from build123d import *

# Parameters (mm, degrees)
F1_DEPTH = 25


with BuildPart() as f1:
    # F0 (on Front) → F1 (new body)
    with BuildSketch(Plane.XZ):
        with BuildLine():
            ThreePointArc((0.492404, 26.751671), (0, 27.164847), (-0.492404, 26.751671))
            Line((-0.492404, 26.751671), (-4.482871, 4.120605))
            ThreePointArc((-4.482871, 4.120605), (-4.605972, 4.017311), (-4.729073, 4.120605))
            Line((-4.729073, 4.120605), (-8.719541, 26.751671))
            ThreePointArc((-8.719541, 26.751671), (-9.211945, 27.164847), (-9.704349, 26.751671))
            Line((-9.704349, 26.751671), (-14.42139, 0))
            Line((-14.42139, 0), (-13.451544, 0))
            Line((-13.451544, 0), (-9.365199, 23.17481))
            ThreePointArc((-9.365199, 23.17481), (-9.242099, 23.278104), (-9.118998, 23.17481))
            Line((-9.118998, 23.17481), (-5.109237, 0.434329))
            ThreePointArc((-5.109237, 0.434329), (-4.945978, 0.126497), (-4.621282, 5.9e-05))
            ThreePointArc((-4.621282, 5.9e-05), (-4.304656, 0.119468), (-4.136591, 0.413176))
            Line((-4.136591, 0.413176), (-4.105972, 0.586824))
            Line((-4.105972, 0.586824), (-0.123101, 23.17481))
            ThreePointArc((-0.123101, 23.17481), (0, 23.278104), (0.123101, 23.17481))
            Line((0.123101, 23.17481), (4.209445, 0))
            Line((4.209445, 0), (5.209445, 0))
            Line((5.209445, 0), (0.492404, 26.751671))
        make_face()
    extrude(amount=F1_DEPTH)


solid = f1.part
The model under review builds one solid part; all positions refer to its coordinate system, in mm. A direction names the side the tool comes from. Coordinates: 2 decimals unless noted, no trailing zeros. Loops run counter-clockwise (first coordinate to the right, second up) from the corner with the lowest first, then second, coordinate; pieces in that order, holes last. Notation, with made-up numbers: (-14, -15.75) -> (18, -15.75) arc R16 cw to (18, 0.25) -> close; hole circle Ø9 at (31, 59.25). An arc over 180 degrees is marked (long way). Use a Markdown table: item, result. Add a question column.
1. Add section B-B on y = -8.5. Write out the cut boundary in (x, z) (3 decimals), plus the area to 3 significant figures.
2. Add section C-C on x = 2.25. Write out the cut boundary in (y, z), plus the area to 3 significant figures.
3. Machinability: for faces 4 (the face through (-14, -12, 0)), 5 (the face through (-7.14, -12.32, 11.96)), 6 (the face through (-6.7, -12.3, 15.3)), which of the approach directions +Z, -Z, +X, -X, +Y, -Y give a long, thin tool a straight path to every point of the face, cutting with its end or side? Answer none if there is none.
4. Add section D-D on x = -7.5. Write out the cut boundary in (y, z).
5. To check wall thickness, follow line 1 (X direction, y = -11.75, z = 18.75); line 2 (X direction, y = -6.25, z = 8.5); line 3 (Z direction, x = -9.25, y = -1.25). State the ranges of each line that lie inside material, in increasing order.
6. Clearance check with flat-ended pins moving along their axes: pin 1 Ø12 at (y, z) = (-11, 21.5) entering from +X; pin 2 Ø4 at (y, z) = (-16, 13.5) entering from +X; pin 3 Ø1 at (y, z) = (-16.5, 4.5) entering from +X. State where each tip first meets the part, or that it passes through.
7. Add section A-A on z = 2.25. Write out the cut boundary in (x, y), plus the area to 3 significant figures.
8. Draft analysis for pull direction X (two halves, no side actions). For faces 1 (the face through (-12.03, -12.32, 13.56)), 2 (the face through (-11.437, -12.325, 11.425)), 3 (the face through (-7, -25, 14)), state which applies: pulls with the +X half, pulls with the -X half, needs draft (parallel to the pull), parting line crosses it, or undercut.
Returned:
| question | item | result |
|---|---|---|
| 1 | outline | (-14.421, 0) -> (-13.452, 0) -> (-9.365, 23.175) arc R0.125 cw to (-9.119, 23.175) -> (-5.109, 0.434) arc R0.5 ccw to (-4.621, 0) arc R0.5 ccw to (-4.137, 0.413) -> (-4.106, 0.587) -> (-0.123, 23.175) arc R0.125 cw to (0.123, 23.175) -> (4.209, 0) -> (5.209, 0) -> (0.492, 26.752) arc R0.5 ccw to (-0.492, 26.752) -> (-4.483, 4.121) arc R0.125 cw to (-4.729, 4.121) -> (-8.72, 26.752) arc R0.5 ccw to (-9.704, 26.752) -> close |
| 1 | area | 103 mm² |
| 2 | outline | (-25, 11.11) -> (0, 11.11) -> (0, 16.78) -> (-25, 16.78) -> close |
| 2 | area | 142 mm² |
| 3 | face 4 | -Z, +X, -X, +Y, -Y |
| 3 | face 5 | -Z, +Y, -Y |
| 3 | face 6 | +Z, +Y, -Y |
| 4 | outline | (-25, 13.99) -> (0, 13.99) -> (0, 19.84) -> (-25, 19.84) -> close |
| 5 | line 1 | x = -11.12 to -10.15, -8.34 to -7.31, -1.9 to -0.9, 0.9 to 1.9 |
| 5 | line 2 | x = -12.92 to -11.95, -6.53 to -5.5, -3.71 to -2.71, 2.71 to 3.71 |
| 5 | line 3 | z = 23.28 to 27.16 |
| 6 | pin 1 | stops at x = 2.48 |
| 6 | pin 2 | stops at x = 3.18 |
| 6 | pin 3 | stops at x = 4.5 |
| 7 | outline | (-14.02, -25) -> (-13.05, -25) -> (-13.05, 0) -> (-14.02, 0) -> close; (-5.43, -25) -> (-3.81, -25) -> (-3.81, 0) -> (-5.43, 0) -> close; (3.81, -25) -> (4.81, -25) -> (4.81, 0) -> (3.81, 0) -> close |
| 7 | area | 89.7 mm² |
| 8 | face 1 | pulls with the -X half |
| 8 | face 2 | undercut |
| 8 | face 3 | needs draft |
